Verification items for the finished model (mm, model axes). A direction names the side the tool comes from. Round coordinates to 2 decimals unless told otherwise and drop trailing zeros. Loops run counter-clockwise (first coordinate to the right, second up) from the corner with the lowest first, then second, coordinate; pieces in that order, holes last.
from build123d import *

# Parameters (mm, degrees)
SKETCH1_W           = 76
SKETCH1_H           = 96
SKETCH1_W_2         = 30
SKETCH1_H_2         = 40
BOSS_EXTRUDE1_DEPTH = 0.25
SKETCH2_W           = 76
SKETCH2_H           = 96
BOSS_EXTRUDE2_DEPTH = 4
SKETCH3_W           = 30
SKETCH3_H           = 40
CUT_EXTRUDE1_DEPTH  = 0.25
SKETCH4_W           = 30
SKETCH4_H           = 40
CUT_EXTRUDE2_DEPTH  = 0.5
SKETCH5_W           = 30
SKETCH5_H           = 40
CUT_EXTRUDE3_DEPTH  = 0.75
SKETCH6_W           = 83.006350466
SKETCH6_H           = 7.589152043
CUT_EXTRUDE4_DEPTH  = 107.75


with BuildPart() as part:
    # Sketch1 → Boss-Extrude1 (new body)
    with BuildSketch(Plane(origin=(0, 0, 0), x_dir=(1, 0, 0), z_dir=(0, 1, 0))):
        Rectangle(SKETCH1_W, SKETCH1_H)
        with Locations((-18, 23)):
            Rectangle(SKETCH1_W_2, SKETCH1_H_2, mode=Mode.SUBTRACT)
        with Locations((18, 23)):
            Rectangle(SKETCH1_W_2, SKETCH1_H_2, mode=Mode.SUBTRACT)
        with Locations((18, -23)):
            Rectangle(SKETCH1_W_2, SKETCH1_H_2, mode=Mode.SUBTRACT)
        with Locations((-18, -23)):
            Rectangle(SKETCH1_W_2, SKETCH1_H_2, mode=Mode.SUBTRACT)
    extrude(amount=BOSS_EXTRUDE1_DEPTH)

    # Sketch2 → Boss-Extrude2 (add)
    with BuildSketch(Plane.XZ):
        Rectangle(SKETCH2_W, SKETCH2_H)
    extrude(amount=BOSS_EXTRUDE2_DEPTH)

    # Sketch3 → Cut-Extrude1 (cut)
    with BuildSketch(Plane(origin=(0, 0, 0), x_dir=(1, 0, 0), z_dir=(0, 1, 0))):
        with Locations((-18, 23)):
            Rectangle(SKETCH3_W, SKETCH3_H)
    extrude(amount=-CUT_EXTRUDE1_DEPTH, mode=Mode.SUBTRACT)

    # Sketch4 → Cut-Extrude2 (cut)
    with BuildSketch(Plane(origin=(0, 0, 0), x_dir=(1, 0, 0), z_dir=(0, 1, 0))):
        with Locations((18, -23)):
            Rectangle(SKETCH4_W, SKETCH4_H)
    extrude(amount=-CUT_EXTRUDE2_DEPTH, mode=Mode.SUBTRACT)

    # Sketch5 → Cut-Extrude3 (cut)
    with BuildSketch(Plane(origin=(0, 0, 0), x_dir=(1, 0, 0), z_dir=(0, 1, 0))):
        with Locations((18, 23)):
            Rectangle(SKETCH5_W, SKETCH5_H)
    extrude(amount=-CUT_EXTRUDE3_DEPTH, mode=Mode.SUBTRACT)

    # Sketch6 → Cut-Extrude4 (cut)
    with BuildSketch(Plane.XY.offset(48)):
        with Locations((-0.355741502, -6.544576022)):
            Rectangle(SKETCH6_W, SKETCH6_H)
    extrude(amount=-CUT_EXTRUDE4_DEPTH, mode=Mode.SUBTRACT)


solid = part.part
1. Scan lines: L1, parallel to Z at x = 5, y = -0.2; L2, parallel to X at y = 0, z = -6.5; L3, parallel to X at y = -0.3, z = -37.5. Record each from-to range of solid material in increasing order.
2. Section check A-A (x = 22.5). Enter the section's corners in (y, z).
3. Section check B-B (z = 42). Enter the section's corners in (x, y), then the cut area to 3 significant figures.
4. Tool access check on faces 4 (the face through (18, -0.5, 23)), 5 (the face through (38, -1, -1)). Record the directions out of +Z, -Z, +X, -X, +Y, -Y that give a thin tool (end or side, any length) a straight path to the whole face; none if there is none.
5. Release check for a two-part mould opening along X. For faces 1 (the face through (-38, -1, -1)), 2 (the face through (-1, -1, -48)), 3 (the face through (-18, -0.25, -23)) record: released by +X, released by -X, zero draft, split by the parting line, or undercut.
6. Gauge pin test, flat ends, axial feed: P1, Ø8, axis at x = 11.5, z = -26.5, coming from the +Y side; P2, Ø24, axis at x = -17, z = -19.5, coming from the +Y side. Record the tip position at first contact, or that the pin passes through.
Taken from the geometry:
1. L1: z = -48 to -43, -3 to 3, 43 to 48
1. L2: x = -38 to -33, -3 to 3, 33 to 38
1. L3: x = -38 to 3, 33 to 38
2. outline: (-2.75, -48) - (0.25, -48) - (0.25, -43) - (-0.75, -43) - (-0.75, -3) - (0.25, -3) - (0.25, 3) - (-0.5, 3) - (-0.5, 43) - (0.25, 43) - (0.25, 48) - (-2.75, 48) - close
3. outline: (-38, -2.75) - (38, -2.75) - (38, 0.25) - (33, 0.25) - (33, -0.5) - (3, -0.5) - (3, 0.25) - (-3, 0.25) - (-3, 0) - (-33, 0) - (-33, 0.25) - (-38, 0.25) - close
3. area: 198 mm2
4. face 4: +Y
4. face 5: +Z, -Z, +X, +Y, -Y
5. face 1: released by -X
5. face 2: zero draft
5. face 3: undercut
6. P1: stops at y = -0.75
6. P2: stops at y = -0.25
